```python
from build123d import *

# Parameters (mm, degrees)
PAD_DEPTH           = 45.72
PAD_DEPTH_BACK      = 45.72
SKETCH001_W         = 2.032
SKETCH001_H         = 20.32
POCKET_DEPTH        = 53.341
SKETCH002_W         = 6
SKETCH002_H         = 71.374
PAD001_DEPTH        = 2.54
PAD001_DEPTH_BACK   = 2.54
SKETCH003_R         = 1.7
HOLE_DEPTH          = 5.081
SKETCH004_W         = 6
SKETCH004_H         = 71.374
PAD002_DEPTH        = 7.62
HOLE001_D           = 3.4
HOLE001_DEPTH       = 24.892
HOLE001_CBORE_D     = 6.1
HOLE001_CBORE_DEPTH = 3.302
CHAMFER_SIZE2       = 7.366
CHAMFER_SIZE        = 2.032


with BuildPart() as part:
    # Sketch → Pad (new body, two sides)
    with BuildSketch(Plane.YZ) as pad_sk:
        Polygon((-26.67, 21.59), (-26.67, 0), (26.67, 0), (26.67, 21.59), (24.13, 21.59), (24.13, 2.54), (1.27, 2.54), (1.27, 21.59), (-1.27, 21.59), (-1.27, 2.54), (-24.13, 2.54), (-24.13, 21.59), align=None)
    extrude(amount=PAD_DEPTH)
    extrude(pad_sk.sketch, amount=-PAD_DEPTH_BACK)

    # Sketch001 (on Face1 of Pad) → Pocket (cut, through all)
    with BuildSketch(Plane(origin=(0, -26.67, 0), x_dir=(0, 0, -1), z_dir=(0, -1, 0))):
        with Locations((-18.034, -22.86)):
            Rectangle(SKETCH001_W, SKETCH001_H)
        with Locations((-18.034, 22.86)):
            Rectangle(SKETCH001_W, SKETCH001_H)
    extrude(amount=-POCKET_DEPTH, mode=Mode.SUBTRACT)

    # Sketch002 (on Face5 of Pocket) → Pad001 (join, two sides)
    with BuildSketch(Plane.YX) as pad001_sk:
        with Locations((-29.67, 0)):
            Rectangle(SKETCH002_W, SKETCH002_H)
    extrude(amount=-PAD001_DEPTH)
    extrude(pad001_sk.sketch, amount=PAD001_DEPTH_BACK)

    # Sketch003 (on Face5 of Pad001) → Hole (cut, through all)
    with BuildSketch(Plane(origin=(0, 0, 2.54), x_dir=(0, -1, 0), z_dir=(0, 0, 1))):
        with Locations((29.67, -24.892)):
            Circle(SKETCH003_R)
        with Locations((29.67, 24.892)):
            Circle(SKETCH003_R)
    extrude(amount=-HOLE_DEPTH, mode=Mode.SUBTRACT)

    # Sketch004 (on Face3 of Hole) → Pad002 (join)
    with BuildSketch(Plane.YX):
        with Locations((13.51, 0)):
            Rectangle(SKETCH004_W, SKETCH004_H)
    extrude(amount=PAD002_DEPTH)

    # Hole001
    with Locations(Plane(origin=(0, 0, 2.54), x_dir=(0, -1, 0), z_dir=(0, 0, 1))):
        with Locations((-13.51, 24.892), (-13.51, -24.892)):
            CounterBoreHole(HOLE001_D / 2, HOLE001_CBORE_D / 2, HOLE001_CBORE_DEPTH, depth=HOLE001_DEPTH)

    # Chamfer
    chamfer_edges = [part.edges().sort_by_distance(p)[0] for p in [
        (-40.7035, -26.67, 0),
        (40.7035, -26.67, 0),
    ]]
    chamfer_side = part.faces().sort_by_distance((0, -26.67, 11.455103))[0]
    chamfer(chamfer_edges, length=CHAMFER_SIZE, length2=CHAMFER_SIZE2, reference=chamfer_side)


solid = part.part
```
Read the model definition and answer for the solid it produces. Units are mm, in the model's axes. A direction names the side the tool comes from. Round coordinates to 2 decimals unless told otherwise and drop trailing zeros. Write each loop counter-clockwise with the first axis right and the second up, starting at its lowest first coordinate (ties: lowest second). Pieces come first, ordered by that corner, then holes. Notation, with made-up numbers: (55.25, -15) - (108.25, -15) arc R8 ccw to (108.25, -5) - close; hole circle Ø4 at (-28.5, -7.75). An arc over 180 degrees is marked (long way). Use CSV: the item, a comma, the result in double quotes.
Q1. Find section D-D, the plane y = 13.51. Write down the section's boundary in (x, z), then the cut area to 3 significant figures.
Values:
outline,"(-45.72, 0) - (-35.69, 0) - (-35.69, -7.62) - (-26.59, -7.62) - (-26.59, -0.76) - (-27.94, -0.76) - (-27.94, 2.54) - (-45.72, 2.54) - close; (-23.19, -7.62) - (23.19, -7.62) - (23.19, -0.76) - (21.84, -0.76) - (21.84, 2.54) - (-21.84, 2.54) - (-21.84, -0.76) - (-23.19, -0.76) - close; (26.59, -7.62) - (35.69, -7.62) - (35.69, 0) - (45.72, 0) - (45.72, 2.54) - (27.94, 2.54) - (27.94, -0.76) - (26.59, -0.76) - close"
area,"689 mm²"
Q2. Find section B-B, the plane x = -40. Write down the section's boundary in (y, z).
Values:
outline,"(-26.67, 2.03) - (-19.3, 0) - (26.67, 0) - (26.67, 21.59) - (24.13, 21.59) - (24.13, 2.54) - (1.27, 2.54) - (1.27, 21.59) - (-1.27, 21.59) - (-1.27, 2.54) - (-24.13, 2.54) - (-24.13, 21.59) - (-26.67, 21.59) - close"
Q3. Determine the mould class of faces 5 (the flat face through (0, 13, -7.62)), 6 (the cylindrical face through (25.8, 10.6, 0.9)), 7 (the flat face through (-33.02, 25, 18)), 8 (the flat face through (45.72, 0, 6)) for opening direction X: +X half, -X half, draft (parallel to the pull), parting line (faces both ways), or undercut.
Values:
face 5,"draft"
face 6,"undercut"
face 7,"undercut"
face 8,"+X half"
Q4. Straight lines are drawn through the part: line 1 along X through (y, z) = (13.51, -3); line 2 along Y through (x, z) = (30.5, 10); line 3 along X through (y, z) = (-0.5, 18). For each, find the intervals that lie inside material, in ascending order.
Values:
line 1,"x = -35.69 to -26.59, -23.19 to 23.19, 26.59 to 35.69"
line 2,"y = -26.67 to -24.13, -1.27 to 1.27, 24.13 to 26.67"
line 3,"x = -45.72 to -33.02, -12.7 to 12.7, 33.02 to 45.72"
Q5. A tool of negligible diameter and unlimited length cuts with its end or side. For faces 1 (the flat face through (0, 16.51, -4)), 2 (the flat face through (1, 1.27, 12)), 3 (the flat face through (-26, 12, -0.762)), 4 (the flat face through (-12.7, -25, 18)), from which of +Z, -Z, +X, -X, +Y, -Y can it reach the whole face along a straight path? Write none if from no direction.
Values:
face 1,"-Z, +X, -X, +Y"
face 2,"+Z, +X, -X"
face 3,"+Z"
face 4,"+Y, -Y"
Q6. Each of these flat-tipped pins is pushed along its axis until it touches: pin 1 Ø5 at (x, y) = (-1.5, -30.5) entering from -Z; pin 2 Ø5 at (x, z) = (-18.5, 9.5) entering from -Y; pin 3 Ø1.3 at (x, y) = (-20.5, -25) entering from -Z; pin 4 Ø4 at (y, z) = (4.5, 6.5) entering from -X. Where does it stop, or does it pass through?
Values:
pin 1,"stops at z = -2.54"
pin 2,"stops at y = -26.67"
pin 3,"stops at z = 0"
pin 4,"passes through"
Q7. Find section A-A, the plane y = -29.67. Write down the section's boundary in (x, z), then the cut area to 3 significant figures.
Values:
outline,"(-35.69, -2.54) - (-26.59, -2.54) - (-26.59, 2.54) - (-35.69, 2.54) - close; (-23.19, -2.54) - (23.19, -2.54) - (23.19, 2.54) - (-23.19, 2.54) - close; (26.59, -2.54) - (35.69, -2.54) - (35.69, 2.54) - (26.59, 2.54) - close"
area,"328 mm²"
Q8. Find section C-C, the plane x = 17.5. Count the separate pieces of the cut face and the enclosed holes in it, then the cut area to 3 significant figures.
Values:
separate pieces,"4"
enclosed holes,"0"
area,"341 mm²"
